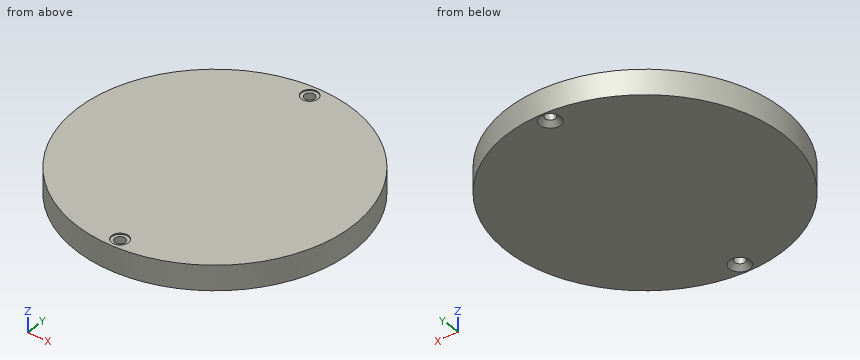
from build123d import *

# Parameters (mm, degrees)
SKETCH1_R           = 36
BOSS_EXTRUDE1_DEPTH = 6.5
SKETCH11_R          = 2.1844
CUT_EXTRUDE3_DEPTH  = 0.3


with BuildPart() as part:
    # Sketch1 → Boss-Extrude1 (new body)
    with BuildSketch(Plane.XY):
        with Locations(Location((0, 0, 0), (0, 0, 180))):
            Circle(SKETCH1_R)
    extrude(amount=BOSS_EXTRUDE1_DEPTH)

    # Sketch10 → #4-40 Tapped Hole1 (revolve, cut)
    with BuildSketch(Plane(origin=(0, -33, 0), x_dir=(0, 1, 0), z_dir=(1, 0, 0))):
        Polygon((0, 0), (0, 7.311161816), (1.349999967, 6.5), (1.349999967, 1.132779999), (2.6999946, 0), align=None)
    f_4_40_tapped_hole1 = revolve(axis=Axis((0, -33, -6.35), (0, 0, 1)), mode=Mode.SUBTRACT)

    # Sketch11 → Cut-Extrude3 (cut)
    with BuildSketch(Plane.XY.offset(6.5)):
        with Locations((0, -33)):
            Circle(SKETCH11_R)
    cut_extrude3 = extrude(amount=-CUT_EXTRUDE3_DEPTH, mode=Mode.SUBTRACT)

    # Mirror1: #4-40 Tapped Hole1, Cut-Extrude3 across plane
    add(f_4_40_tapped_hole1.mirror(Plane(origin=(0, 0, 0), x_dir=(0, 0, 1), z_dir=(0, -1, 0))), mode=Mode.SUBTRACT)
    add(cut_extrude3.mirror(Plane(origin=(0, 0, 0), x_dir=(0, 0, 1), z_dir=(0, -1, 0))), mode=Mode.SUBTRACT)


solid = part.part
Geometry check sheet. Reference: the model listing, model coordinates, mm. Round coordinates to 2 decimals unless told otherwise and drop trailing zeros. Loops run counter-clockwise (first coordinate to the right, second up) from the corner with the lowest first, then second, coordinate; pieces in that order, holes last.
Item 1: Gauge pin test, flat ends, axial feed: pin 1 (4 mm diameter, centred on x = 0, y = -33, fed in from -Z); pin 2 (1 mm diameter, centred on x = -19.5, y = -6, fed in from -Z); pin 3 (1.3 mm diameter, centred on x = -1, y = 32, fed in from +Z); pin 4 (1 mm diameter, centred on x = -22.5, z = 5.5, fed in from -Y). Record the tip position at first contact, or that the pin passes through.
Item 2: Thickness scan on line 1 (Y direction, x = 0, z = 2.5); line 2 (Y direction, x = 0, z = 6.45); line 3 (X direction, y = 32, z = 2.25). Record the ranges inside material, lowest first.
Item 3: Cross-section at B-B on y = 33. Record the boundary of the cut face in (x, z).
Item 4: Cross-section at C-C on z = 4. Record the boundary of the cut face in (x, y).
Item 5: Cross-section at D-D on x = -32. Record the boundary of the cut face in (y, z), then the cut area to 3 significant figures.
Item 6: Cross-section at A-A on x = 0. Record the boundary of the cut face in (y, z).
Answer sheet:
1. pin 1: stops at z = 0.59
1. pin 2: stops at z = 0
1. pin 3: stops at z = 6.2
1. pin 4: stops at y = -28.5
2. line 1: y = -36 to -34.35, -31.65 to 31.65, 34.35 to 36
2. line 2: y = -36 to -35.18, -30.82 to 30.82, 35.18 to 36
2. line 3: x = -16.49 to -0.91, 0.91 to 16.49
3. outline: (-14.39, 0) - (-2.7, 0) - (-1.35, 1.13) - (-1.35, 6.2) - (-2.18, 6.2) - (-2.18, 6.5) - (-14.39, 6.5) - close; (1.35, 1.13) - (2.7, 0) - (14.39, 0) - (14.39, 6.5) - (2.18, 6.5) - (2.18, 6.2) - (1.35, 6.2) - close
4. outline: circle Ø72 at (0, 0); hole circle Ø2.7 at (0, -33); hole circle Ø2.7 at (0, 33)
5. outline: (-16.49, 0) - (16.49, 0) - (16.49, 6.5) - (-16.49, 6.5) - close
5. area: 214 mm2
6. outline: (-36, 0) - (-35.7, 0) - (-34.35, 1.13) - (-34.35, 6.2) - (-35.18, 6.2) - (-35.18, 6.5) - (-36, 6.5) - close; (-31.65, 1.13) - (-30.3, 0) - (30.3, 0) - (31.65, 1.13) - (31.65, 6.2) - (30.82, 6.2) - (30.82, 6.5) - (-30.82, 6.5) - (-30.82, 6.2) - (-31.65, 6.2) - close; (34.35, 1.13) - (35.7, 0) - (36, 0) - (36, 6.5) - (35.18, 6.5) - (35.18, 6.2) - (34.35, 6.2) - close
